```python
from build123d import *

# Parameters (mm, degrees)
BOSS_EXTRUDE1_DEPTH  = 1.5
SKETCH2_R            = 1.25
CUT_EXTRUDE1_DEPTH   = 19.276094358
SKETCH3_R            = 0.5
CUT_EXTRUDE2_DEPTH   = 19.276094358
LPATTERN1_COUNT      = 10
LPATTERN1_PITCH      = 2.5
SKETCH4_W            = 6
SKETCH4_H            = 5
GAIN_SWITCH_DEPTH    = 3.3
SKETCH5_R            = 0.5
CUT_EXTRUDE3_DEPTH   = 19.510959592
LPATTERN2_COUNT      = 2
LPATTERN2_PITCH      = 3.5
LPATTERN2_COUNT_DIR2 = 2
LPATTERN2_PITCH_DIR2 = 8


with BuildPart() as part:
    # Sketch1 → Boss-Extrude1 (new body)
    with BuildSketch(Plane.XY):
        with BuildLine():
            Line((-10.5, -14.125), (10.5, -14.125))
            ThreePointArc((10.5, -14.125), (11.207106781, -13.832106781), (11.5, -13.125))
            Line((11.5, -13.125), (11.5, 13.125))
            ThreePointArc((11.5, 13.125), (11.207106781, 13.832106781), (10.5, 14.125))
            Line((10.5, 14.125), (-10.5, 14.125))
            ThreePointArc((-10.5, 14.125), (-11.207106781, 13.832106781), (-11.5, 13.125))
            Line((-11.5, 13.125), (-11.5, -13.125))
            ThreePointArc((-11.5, -13.125), (-11.207106781, -13.832106781), (-10.5, -14.125))
        make_face()
    extrude(amount=BOSS_EXTRUDE1_DEPTH)

    # Sketch2 → Cut-Extrude1 (cut, through all)
    with BuildSketch(Plane.XY.offset(1.5)):
        with Locations((9, 11.625)):
            Circle(SKETCH2_R)
    cut_extrude1 = extrude(amount=-CUT_EXTRUDE1_DEPTH, mode=Mode.SUBTRACT)

    # Mirror1: Cut-Extrude1 across plane
    add(cut_extrude1.mirror(Plane.ZX), mode=Mode.SUBTRACT)

    # Sketch3 → Cut-Extrude2 (cut, through all)
    with BuildSketch(Plane.XY.offset(1.5)):
        with Locations((-10, -11.625)):
            Circle(SKETCH3_R)
    cut_extrude2 = extrude(amount=-CUT_EXTRUDE2_DEPTH, mode=Mode.SUBTRACT)

    # LPattern1: Cut-Extrude2 ×10
    with Locations(*[(0, i * LPATTERN1_PITCH, 0) for i in range(1, LPATTERN1_COUNT)]):
        add(cut_extrude2, mode=Mode.SUBTRACT)

    # Sketch4 → Gain Switch (add)
    with BuildSketch(Plane.XY.offset(1.5)):
        with Locations((0, -11.425)):
            Rectangle(SKETCH4_W, SKETCH4_H)
    extrude(amount=GAIN_SWITCH_DEPTH)

    # Sketch5 → Cut-Extrude3 (cut, through all)
    with BuildSketch(Plane.XY.offset(1.5)):
        with Locations((7.7, 6.125)):
            Circle(SKETCH5_R)
    cut_extrude3 = extrude(amount=-CUT_EXTRUDE3_DEPTH, mode=Mode.SUBTRACT)

    # LPattern2: Cut-Extrude3 2 × 2
    with Locations(*[Vector(0, -1, 0) * (i * LPATTERN2_PITCH) + Vector(0, -1, 0) * (j * LPATTERN2_PITCH_DIR2) for i in range(LPATTERN2_COUNT) for j in range(LPATTERN2_COUNT_DIR2) if (i, j) != (0, 0)]):
        add(cut_extrude3, mode=Mode.SUBTRACT)


solid = part.part
```
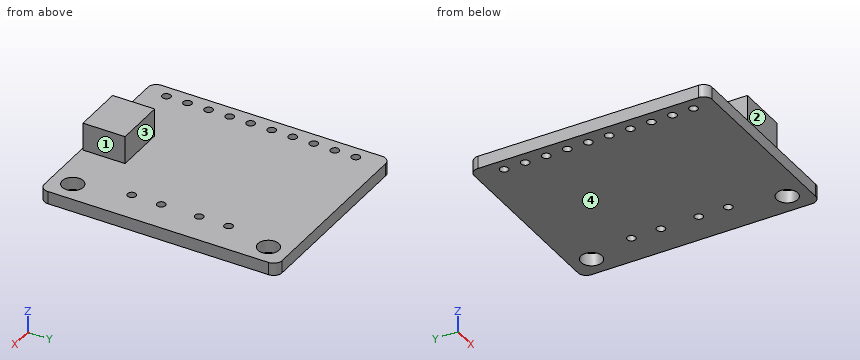
Geometry check sheet. Reference: the model listing, model coordinates, mm. Face numbers are marked on the shaded views. A direction names the side the tool comes from. Round coordinates to 2 decimals unless told otherwise and drop trailing zeros. Loops run counter-clockwise (first coordinate to the right, second up) from the corner with the lowest first, then second, coordinate; pieces in that order, holes last. Notation, with made-up numbers: (-12, 83.5) - (-8, 83.5) arc R37 ccw to (-8, 119.5) - close; hole circle Ø5 at (-3.5, 38.25). An arc over 180 degrees is marked (long way). Write item = value, one per line. Start each with the question number.
1. Section check B-B on z = 1. Give the number of separate pieces and of enclosed holes in the cut face, then the cut area to 3 significant figures.
2. Thickness scan on line 1 (Y direction, x = 7.7, z = 0.5) (3 decimals); line 2 (Y direction, x = 9, z = 0.3) (3 decimals); line 3 (Y direction, x = 10, z = 1.45) (3 decimals). Record the ranges inside material, lowest first.
3. Set-up check for the marked faces 1, 2, 3 and 4: record each of +Z, -Z, +X, -X, +Y, -Y from which the full face is reachable in a straight line by a thin tool's end or side.
4. Depth check by flat-ended pin: pin 1 (2 mm diameter, centred on x = 9, y = -11.625, fed in from +Z); pin 2 (2.5 mm diameter, centred on y = -12, z = 3, fed in from +X); pin 3 (8 mm diameter, centred on x = 1, y = 0.5, fed in from -Z); pin 4 (7 mm diameter, centred on x = 0.5, y = 3.5, fed in from +Z). Enter the tip coordinate at first touch or a pass-through.
5. Section check A-A on x = 9. Enter the section's corners in (y, z) (3 decimals).
6. Section check D-D on z = 4.25. Enter the section's corners in (x, y) (3 decimals), then the cut area to 3 significant figures.
Working result:
q1.separate_pieces = 1
q1.enclosed_holes = 16
q1.area = 628 mm^2
q2.line_1 = -14.125 to -5.875, -4.875 to -2.375, -1.375 to 2.125, 3.125 to 5.625, 6.625 to 14.125
q2.line_2 = -14.125 to -12.875, -10.375 to 10.375, 12.875 to 14.125
q2.line_3 = -14.125 to -12.375, -10.875 to 10.875, 12.375 to 14.125
q3.face_1 = +Z, +X, +Y, -Y
q3.face_2 = +Z, +X, -X, -Y
q3.face_3 = +Z, +X, -X, +Y
q3.face_4 = -Z, +X, -X, +Y, -Y
q4.pin_1 = through
q4.pin_2 = 3
q4.pin_3 = 0
q4.pin_4 = 1.5
q5.outline = (-14.125, 0) - (-12.875, 0) - (-12.875, 1.5) - (-14.125, 1.5) - close; (-10.375, 0) - (10.375, 0) - (10.375, 1.5) - (-10.375, 1.5) - close; (12.875, 0) - (14.125, 0) - (14.125, 1.5) - (12.875, 1.5) - close
q6.outline = (-3, -13.925) - (3, -13.925) - (3, -8.925) - (-3, -8.925) - close
q6.area = 30.0 mm^2
